from build123d import *

# Parameters (mm, degrees)
BOX116_W          = 56
BOX116_H          = 37
BOX116_DEPTH      = 6
BOX130_W          = 60
BOX130_H          = 30
BOX130_DEPTH      = 6
CYLINDER224_R     = 1.5
CYLINDER224_DEPTH = 12
BOX131_W          = 12
BOX131_H          = 30
BOX131_DEPTH      = 6
CYLINDER222_R     = 1.5
CYLINDER222_DEPTH = 12
CYLINDER221_R     = 1.5
CYLINDER221_DEPTH = 12
CYLINDER223_R     = 1.5
CYLINDER223_DEPTH = 12
BOX134_W          = 25
BOX134_H          = 45
BOX134_DEPTH      = 6
BOX097_W          = 100
BOX097_H          = 42
BOX097_DEPTH      = 3
FILLET082_R       = 8


with BuildPart() as obj1:
    # Box116 → Box116 (new body)
    with BuildSketch(Plane(origin=(-38, -18.5, 13), x_dir=(1, 0, 0), z_dir=(0, 0, 1))):
        with Locations((28, 18.5)):
            Rectangle(BOX116_W, BOX116_H)
    extrude(amount=BOX116_DEPTH)


with BuildPart() as obj2:
    # Box130 → Box130 (new body)
    with BuildSketch(Plane(origin=(-42, -15, 13), x_dir=(1, 0, 0), z_dir=(0, 0, 1))):
        with Locations((30, 15)):
            Rectangle(BOX130_W, BOX130_H)
    extrude(amount=BOX130_DEPTH)


with BuildPart() as zylinder224:
    # Cylinder224 → Cylinder224 (new body)
    with BuildSketch(Plane(origin=(25.5, 17.5, 8), x_dir=(1, 0, 0), z_dir=(0, 0, 1))):
        Circle(CYLINDER224_R)
    extrude(amount=CYLINDER224_DEPTH)


with BuildPart() as obj3:
    # Box131 → Box131 (new body)
    with BuildSketch(Plane(origin=(20, -15, 13), x_dir=(1, 0, 0), z_dir=(0, 0, 1))):
        with Locations((6, 15)):
            Rectangle(BOX131_W, BOX131_H)
    extrude(amount=BOX131_DEPTH)


with BuildPart() as zylinder222:
    # Cylinder222 → Cylinder222 (new body)
    with BuildSketch(Plane(origin=(-40.5, -17.5, 8), x_dir=(1, 0, 0), z_dir=(0, 0, 1))):
        Circle(CYLINDER222_R)
    extrude(amount=CYLINDER222_DEPTH)


with BuildPart() as zylinder221:
    # Cylinder221 → Cylinder221 (new body)
    with BuildSketch(Plane(origin=(-40.5, 17.5, 8), x_dir=(1, 0, 0), z_dir=(0, 0, 1))):
        Circle(CYLINDER221_R)
    extrude(amount=CYLINDER221_DEPTH)


with BuildPart() as zylinder223:
    # Cylinder223 → Cylinder223 (new body)
    with BuildSketch(Plane(origin=(25.5, -17.5, 8), x_dir=(1, 0, 0), z_dir=(0, 0, 1))):
        Circle(CYLINDER223_R)
    extrude(amount=CYLINDER223_DEPTH)


with BuildPart() as fusion142:
    # Box134 → Box134 (new body)
    with BuildSketch(Plane(origin=(-70, -22.5, 13), x_dir=(1, 0, 0), z_dir=(0, 0, 1))):
        with Locations((12.5, 22.5)):
            Rectangle(BOX134_W, BOX134_H)
    extrude(amount=BOX134_DEPTH)

    # Fusion142: union obj1, obj2, Zylinder224, obj3, Zylinder222, Zylinder221, Zylinder223
    add(obj1.part)
    add(obj2.part)
    add(zylinder224.part)
    add(obj3.part)
    add(zylinder222.part)
    add(zylinder221.part)
    add(zylinder223.part)


with BuildPart() as cut097:
    # Box097 → Box097 (new body)
    with BuildSketch(Plane(origin=(-68.25, -21, 14), x_dir=(1, 0, 0), z_dir=(0, 0, 1))):
        with Locations((50, 21)):
            Rectangle(BOX097_W, BOX097_H)
    extrude(amount=BOX097_DEPTH)

    # Fillet082
    fillet082_edges = [cut097.edges().sort_by_distance(p)[0] for p in [
        (-68.25, -21, 15.5),
        (-68.25, 21, 15.5),
        (31.75, -21, 15.5),
        (31.75, 21, 15.5),
    ]]
    fillet(fillet082_edges, radius=FILLET082_R)

    # Cut097: cut Fusion142
    add(fusion142.part, mode=Mode.SUBTRACT)


solid = cut097.part
Model file for the job. Use its own axes, mm. A direction names the side the tool comes from. Give positions to 0.01 mm unless a question says otherwise; leave off trailing zeros. Loops run counter-clockwise (first coordinate to the right, second up) from the corner with the lowest first, then second, coordinate; pieces in that order, holes last. Notation, with made-up numbers: (-17.5, -15) - (7.5, -15) arc R9 cw to (7.5, -7) - close; hole circle Ø9 at (-28.75, 25). An arc over 180 degrees is marked (long way). Use one line per item in the form item = value.
(1) Pull direction Y, two halves, no side cores. Call faces 4 (the face through (-11, 21, 15)), 5 (the face through (-7, -19, 17)), 6 (the face through (-10, 18.5, 15)), 7 (the face through (-11, -21, 15)): pulls with the +Y half, pulls with the -Y half, needs draft (parallel to the pull), parting line crosses it, or undercut.
Determined:
face_4 = pulls with the +Y half
face_5 = needs draft
face_6 = undercut
face_7 = pulls with the -Y half
(2) 3-axis set-ups, long thin cutter, end or side, ignore diameter. For faces 1 (the face through (26, 15, 15)), 2 (the face through (-40, 15, 15)), 3 (the face through (28.707, 19.279, 15.521)): which of +Z, -Z, +X, -X, +Y, -Y reach the whole face in a straight line?
Determined:
face_1 = +Z, -Z, +X
face_2 = +Z, -Z
face_3 = +Z, -Z, +X, +Y
(3) Drop flat-ended pins along their axis: P1, Ø3.5, axis at x = -40.5, y = -17.5, coming from the -Z side; P2, Ø1.5, axis at y = 4.5, z = 16, coming from the +X side; P3, Ø1.5, axis at x = 26.5, z = 16, coming from the -Y side; P4, Ø0.9, axis at y = 16, z = 15.5, coming from the +X side. Give the stop position or say it passes through.
Determined:
P1 = 14
P2 = 20
P3 = -20.75
P4 = 31.33
(4) Cut at C-C (z = 16.1). Give the cut face in (x, y), then the cut area to 3 significant figures.
Determined:
outline = (-45, -21) - (23.75, -21) arc R8 ccw to (31.5, -15) - (20, -15) - (20, 15) - (31.5, 15) arc R8 ccw to (23.75, 21) - (-45, 21) - close; hole circle Ø3 at (-40.5, -17.5); hole (-42, -15) - (-38, -15) - (-38, -18.5) - (18, -18.5) - (18, 18.5) - (-38, 18.5) - (-38, 15) - (-42, 15) - close; hole circle Ø3 at (-40.5, 17.5); hole circle Ø3 at (25.5, -17.5); hole circle Ø3 at (25.5, 17.5)
area = 624 mm^2
(5) Cut at D-D (y = 17.5). Give the cut face in (x, z), then the cut area to 3 significant figures.
Determined:
outline = (-45, 14) - (-42, 14) - (-42, 17) - (-45, 17) - close; (-39, 14) - (-38, 14) - (-38, 17) - (-39, 17) - close; (18, 14) - (24, 14) - (24, 17) - (18, 17) - close; (27, 14) - (30.36, 14) - (30.36, 17) - (27, 17) - close
area = 40.1 mm^2
(6) Cut at A-A (x = -30.5). Give the cut face in (y, z).
Determined:
outline = (-21, 14) - (-18.5, 14) - (-18.5, 17) - (-21, 17) - close; (18.5, 14) - (21, 14) - (21, 17) - (18.5, 17) - close
(7) Drill centre lines: L1, parallel to Y at x = -40.5, z = 15.4; L2, parallel to Y at x = 21.5, z = 14.25; L3, parallel to X at y = 2, z = 15.7. Where is each one in solid material? Low to high.
Determined:
L1 = -21 to -19, -16 to -15, 15 to 16, 19 to 21
L2 = -21 to -15, 15 to 21
L3 = -45 to -42, 18 to 20
(8) Cut at B-B (y = 11). Give the cut face in (x, z).
Determined:
outline = (-45, 14) - (-42, 14) - (-42, 17) - (-45, 17) - close; (18, 14) - (20, 14) - (20, 17) - (18, 17) - close
